Here's how the part is built. I have some questions about the finished solid (model axes, mm). A direction names the side the tool comes from. Coordinates: 2 decimals unless noted, no trailing zeros. Loops run counter-clockwise (first coordinate to the right, second up) from the corner with the lowest first, then second, coordinate; pieces in that order, holes last. Notation, with made-up numbers: M 70,-9 L 124,-9 A19 cw 124,25 Z; hole C 72,63.25 d3. An arc over 180 degrees is marked long. Use one line per item in the form item = value. Start each with the question number.
(1) Imagine slicing it at A-A, the plane y = 1. Please give me the cut outline in (x, z).
(2) Will these pins go through, and if not, where does the flat tip stop? P1, Ø1.6, axis at x = -17, z = 1, coming from the +Y side; P2, Ø6.5, axis at y = 2, z = 10, coming from the -X side; P3, Ø0.8, axis at x = 17, z = 0.5, coming from the -Y side.
(3) Thinking about a two-plate mould opening in X: for faces 4 (the cylindrical face through (-22.25, 0.08, 0.74)), 5 (the flat face through (0, 0, 0)), 6 (the cylindrical face through (17.32, 1.08, 0.76)), which applies, +X half, -X half, draft (parallel to the pull), parting line (faces both ways), or undercut?
(4) On a 3-axis mill with a long thin cutter (end or side, diameter ignored), from which of +Z, -Z, +X, -X, +Y, -Y can I reach the whole of each face in a straight line? I mean faces 1 (the flat face through (-1, 0, 1.5)), 2 (the flat face through (-17, 3.75, 1)), 3 (the flat face through (17, -1, 1.5)). Say none if no direction works.
(5) Imagine slicing it at D-D, the plane x = -1. Please give me the cut outline in (y, z), and give its area (3 significant figures).
(6) Imagine slicing it at C-C, the plane y = -5.5. Please give me the cut outline in (x, z), and give its area (3 significant figures).
(7) Imagine slicing it at B-B, the plane z = 3.25. Please give me the cut outline in (x, y).
(8) Please list where these lines run through material, in increasing order: L1, parallel to Y at x = -18.5, z = 0.9; L2, parallel to X at y = 1, z = 10.5.
```python
from build123d import *

# Parameters (mm, degrees)
BACK_PLATE_DEPTH               = 1.5
DETECTOR_START                 = 14.75
SKETCH2_W                      = 21.6
SKETCH2_H                      = 13
DETECTOR_SIDE_DEPTH            = 10.45
EMITTER_START                  = -14.75
SKETCH2_2_W                    = 21.6
SKETCH2_2_H                    = 13
EMITTER_SIDE_DEPTH             = 8.95
F_3_2_3_2_DIAMETER_HOLE1_D     = 3.2
F_3_2_3_2_DIAMETER_HOLE1_DEPTH = 4
F_3_2_3_2_DIAMETER_HOLE1_TIP   = 0.96137699


with BuildPart() as part:
    # Sketch1 → Back Plate (new body)
    with BuildSketch(Plane.XY):
        with BuildLine():
            ThreePointArc((-18.5, -3.75), (-15.848349571, -2.651650429), (-14.75, 0))
            ThreePointArc((-14.75, 0), (-15.848349571, 2.651650429), (-18.5, 3.75))
            Line((-18.5, 3.75), (-18.5, -3.75))
        make_face()
        with BuildLine():
            ThreePointArc((-18.5, 3.75), (-22.25, 0), (-18.5, -3.75))
            Line((-18.5, -3.75), (-18.5, 3.75))
        make_face()
        with BuildLine():
            ThreePointArc((-18.5, 3.75), (-15.848349571, 2.651650429), (-14.75, 0))
            Line((-14.75, 0), (-14.75, 3.75))
            Line((-14.75, 3.75), (-18.5, 3.75))
        make_face()
        with BuildLine():
            Line((-18.5, -3.75), (-14.75, -3.75))
            Line((-14.75, -3.75), (-14.75, 0))
            ThreePointArc((-14.75, 0), (-15.848349571, -2.651650429), (-18.5, -3.75))
        make_face()
        Polygon((-14.75, -3.75), (-14.75, -6.5), (14.75, -6.5), (14.75, -3.75), (14.75, 4e-09), (14.75, 3.75), (14.75, 6.5), (-14.75, 6.5), (-14.75, 3.75), (-14.75, 0), align=None)
        with BuildLine():
            Line((14.75, 4e-09), (14.75, -3.75))
            Line((14.75, -3.75), (18.5, -3.75))
            ThreePointArc((18.5, -3.75), (15.848349569, -2.651650428), (14.75, 4e-09))
        make_face()
        with BuildLine():
            Line((14.75, 3.75), (14.75, 4e-09))
            ThreePointArc((14.75, 4e-09), (15.848349572, 2.651650431), (18.5, 3.75))
            Line((18.5, 3.75), (14.75, 3.75))
        make_face()
        with BuildLine():
            ThreePointArc((18.5, 3.75), (15.848349572, 2.651650431), (14.75, 4e-09))
            ThreePointArc((14.75, 4e-09), (15.848349569, -2.651650428), (18.5, -3.75))
            Line((18.5, -3.75), (18.5, 3.75))
        make_face()
        with BuildLine():
            Line((18.5, 3.75), (18.5, -3.75))
            ThreePointArc((18.5, -3.75), (21.151650429, -2.651650429), (22.25, 0))
            ThreePointArc((22.25, 0), (21.151650429, 2.651650429), (18.5, 3.75))
        make_face()
    extrude(amount=BACK_PLATE_DEPTH)

    # Sketch2 → Detector Side (add)
    with BuildSketch(Plane(origin=(0, 0, 0), x_dir=(0, 0, -1), z_dir=(1, 0, 0)).offset(DETECTOR_START)):
        with Locations((-12.3, 0)):
            Rectangle(SKETCH2_W, SKETCH2_H)
    extrude(amount=-DETECTOR_SIDE_DEPTH)

    # Sketch2<2> → Emitter Side (add)
    with BuildSketch(Plane(origin=(0, 0, 0), x_dir=(0, 0, -1), z_dir=(1, 0, 0)).offset(EMITTER_START)):
        with Locations((-12.3, 0)):
            Rectangle(SKETCH2_2_W, SKETCH2_2_H)
    extrude(amount=EMITTER_SIDE_DEPTH)

    # Ø3.2 (3.2) Diameter Hole1
    with Locations(Plane(origin=(0, 0, 0), x_dir=(-1, 0, 0), z_dir=(0, 0, -1))):
        with Locations((-18.5, 0), (18.5, 0)):
            Hole(F_3_2_3_2_DIAMETER_HOLE1_D / 2, depth=F_3_2_3_2_DIAMETER_HOLE1_DEPTH)
            with Locations((0, 0, -(F_3_2_3_2_DIAMETER_HOLE1_DEPTH + F_3_2_3_2_DIAMETER_HOLE1_TIP / 2))):  # 118° drill point
                Cone(0, F_3_2_3_2_DIAMETER_HOLE1_D / 2, F_3_2_3_2_DIAMETER_HOLE1_TIP, mode=Mode.SUBTRACT)


solid = part.part
```
Answer:
q1.outline = M -22.11,0 L -19.75,0 L -19.75,1.5 L -22.11,1.5 Z; M -17.25,0 L 17.25,0 L 17.25,1.5 L 14.75,1.5 L 14.75,23.1 L 4.3,23.1 L 4.3,1.5 L -5.8,1.5 L -5.8,23.1 L -14.75,23.1 L -14.75,1.5 L -17.25,1.5 Z; M 19.75,0 L 22.11,0 L 22.11,1.5 L 19.75,1.5 Z
q2.P1 = 3.75
q2.P2 = -14.75
q2.P3 = -3.75
q3.face_4 = -X half
q3.face_5 = draft
q3.face_6 = undercut
q4.face_1 = +Z, +Y, -Y
q4.face_2 = +Z, -Z, -X, +Y
q4.face_3 = +Z, +X, +Y, -Y
q5.outline = M -6.5,0 L 6.5,0 L 6.5,1.5 L -6.5,1.5 Z
q5.area = 19.5 mm²
q6.outline = M -14.75,0 L 14.75,0 L 14.75,23.1 L 4.3,23.1 L 4.3,1.5 L -5.8,1.5 L -5.8,23.1 L -14.75,23.1 Z
q6.area = 463 mm²
q7.outline = M -14.75,-6.5 L -5.8,-6.5 L -5.8,6.5 L -14.75,6.5 Z; M 4.3,-6.5 L 14.75,-6.5 L 14.75,6.5 L 4.3,6.5 Z
q8.L1 = -3.75 to -1.6, 1.6 to 3.75
q8.L2 = -14.75 to -5.8, 4.3 to 14.75
